Geometry: final body of the model. Coordinates: model frame, mm. A direction names the side the tool comes from. Round coordinates to 2 decimals unless told otherwise and drop trailing zeros. Write each loop counter-clockwise with the first axis right and the second up, starting at its lowest first coordinate (ties: lowest second). Pieces come first, ordered by that corner, then holes. Notation, with made-up numbers: M -37,-20.5 L -20,-20.5 A23 cw -20,16.5 Z; hole C 85,55.25 d4. An arc over 180 degrees is marked long. Answer as CSV lines item,"result". Start each with the question number.
Q1. Section query C-C on z = 0.35. Output: boundary loops of the cut face in (x, y), and give its area (3 significant figures).
Q2. Reachability of faces 5 (the flat face through (15.2, 3, 2)), 6 (the cylindrical face through (1.203, 11.559, 1.521)) from +Z, -Z, +X, -X, +Y, -Y: full face, straight path, thin tool, end or side. Return the list, or none.
Q3. Section query D-D on y = 3. Output: boundary loops of the cut face in (x, z), and give its area (3 significant figures).
Q4. Section query A-A on x = 14. Output: boundary loops of the cut face in (y, z).
Q5. Ray query, probe 1 along X at (y, z) = (6.35, 1.55); probe 2 along Y at (x, z) = (19.05, 0.75); probe 3 along Y at (x, z) = (10.25, 2.1). Return the intervals inside material, ascending.
Q6. Mould query, pull axis X, two halves, no side actions, for faces 1 (the flat face through (13, 4.25, 2)), 2 (the flat face through (0, 4, 1)), 3 (the flat face through (13, 6, 3)), 4 (the flat face through (10.2, 3, 2)). Classes: pulls with the +X half, pulls with the -X half, needs draft (parallel to the pull), parting line crosses it, or undercut.
Q7. First-contact query: pin 1 (1 mm diameter, centred on y = 11.5, z = 1, fed in from -X). Flat tip, straight axial feed; report the tip coordinate or a pass-through.
Q8. Section query B-B on y = 6.35. Output: boundary loops of the cut face in (x, z).
Autodesk Inventor part; units mm, degrees
ref_plane "YZ Plane" through (0, 0, 0) normal (1, 0, 0) x (0, 1, 0)
ref_plane "XZ Plane" through (0, 0, 0) normal (0, 1, 0) x (-1, 0, 0)
ref_plane "XY Plane" through (0, 0, 0) normal (0, 0, 1) x (1, 0, 0)
sketch "Sketch1" plane through (0, 0, 0) normal (0, 0, 1) x (1, 0, 0)
  line L0 (0, 0) -> (25.4, 0)
  line L1 (25.4, 0) -> (25.4, 12.7)
  line L2 (25.4, 12.7) -> (0, 12.7)
  line L3 (0, 12.7) -> (0, 0)
  dimension "d0" = 25.4
  dimension "d1" = 12.7
extrude "Extrusion1" add sketch "Sketch1" along normal blind 3
fillet "Fillet1" radius 4 2 edges at (0, 12.7, 1.5) (25.4, 12.7, 1.5)
sketch "Sketch2" plane through (0, 0, 3) normal (0, 0, 1) x (1, 0, 0)
  line L0 (21.4, 12.7) -> (4, 12.7)
  line L1 (0, 8.7) -> (0, 0)
  line L2 (25.4, 0) -> (25.4, 8.7)
  line L3 (10.2, 4.25) -> (15.2, 4.25)
  line L4 (15.2, 4.25) -> (15.2, 1.25)
  line L5 (15.2, 1.25) -> (10.2, 1.25)
  line L6 (10.2, 1.25) -> (10.2, 4.25)
  line L7 (0, 0) -> (25.4, 0)
  point P0 (12.7, 12.7)
  point P1 (12.7, 4.25)
  point P2 (12.7, 0)
  point P3 (12.7, 1.25)
  point P4 (6.35, 6.35)
  point P5 (19.05, 6.35)
  dimension "d10" = 5
  dimension "d11" = 3
  dimension "d12" = 1.25
  dimension "d15" = 6.35
  dimension "d16" = 6.35
  dimension "d17" = 6.35
extrude "Extrusion2" cut sketch "Sketch2" against normal through all
hole "Hole1" at (19.05, 6.35, 3) at (6.35, 6.35, 3) direction (0, 0, -1) diameter 4.5 end through all
properties part number "Moving Ramp Holder Base"
Entries:
1,outline,"M 0,0 L 25.4,0 L 25.4,8.7 A4 ccw 21.4,12.7 L 4,12.7 A4 ccw 0,8.7 Z; hole C 6.35,6.35 d4.5; hole M 10.2,1.25 L 15.2,1.25 L 15.2,4.25 L 10.2,4.25 Z; hole C 19.05,6.35 d4.5"
1,area,"269 mm^2"
2,face 5,"+Z, -Z"
2,face 6,"+Z, -Z, -X, +Y"
3,outline,"M 0,0 L 10.2,0 L 10.2,3 L 0,3 Z; M 15.2,0 L 25.4,0 L 25.4,3 L 15.2,3 Z"
3,area,"61.2 mm^2"
4,outline,"M 0,0 L 1.25,0 L 1.25,3 L 0,3 Z; M 4.25,0 L 12.7,0 L 12.7,3 L 4.25,3 Z"
5,probe 1,"x = 0 to 4.1, 8.6 to 16.8, 21.3 to 25.4"
5,probe 2,"y = 0 to 4.1, 8.6 to 12.7"
5,probe 3,"y = 0 to 1.25, 4.25 to 12.7"
6,face 1,"undercut"
6,face 2,"pulls with the -X half"
6,face 3,"needs draft"
6,face 4,"undercut"
7,pin 1,"stops at x = 0.73"
8,outline,"M 0,0 L 4.1,0 L 4.1,3 L 0,3 Z; M 8.6,0 L 16.8,0 L 16.8,3 L 8.6,3 Z; M 21.3,0 L 25.4,0 L 25.4,3 L 21.3,3 Z"
